Part print with two shaded views. Sizes in mm from the minimum x, y, z corner. Round coordinates to 2 decimals unless told otherwise and drop trailing zeros. Loops run counter-clockwise (first coordinate to the right, second up) from the corner with the lowest first, then second, coordinate; pieces in that order, holes last.
(1) Cut at B-B on x = 25. List the corners of the cut face in (y, z), then the cut area to 3 significant figures.
(2) Cut at D-D on z = 18.95. List the corners of the cut face in (x, y) (1 decimal).
(3) Flat gauge pins, fed straight in: pin 1 (6 mm diameter, centred on y = 13, z = 25.5, fed in from -X); pin 2 (6 mm diameter, centred on y = 26, z = 11, fed in from +X); pin 3 (1 mm diameter, centred on y = 9, z = 19, fed in from +X) (1 decimal); pin 4 (17.5 mm diameter, centred on x = 18.5, y = 15.5, fed in from -Z). Where does each tip first touch, or does it go through?
(4) Mould opens along Y. For the marked faces 1 and 2 say: +Y half, -Y half, draft (parallel to the pull), parting line (faces both ways), or undercut.
(5) Cut at A-A on y = 30. List the corners of the cut face in (x, z).
(6) Cut at C-C on z = 31.5. List the corners of the cut face in (x, y).
(7) Probe probe 1 along Y at (x, z) = (30, 11.5); probe 2 along Y at (x, z) = (30, 1); probe 3 along Z at (x, y) = (23.5, 2.5). List the from-to ranges inside material, lowest first.
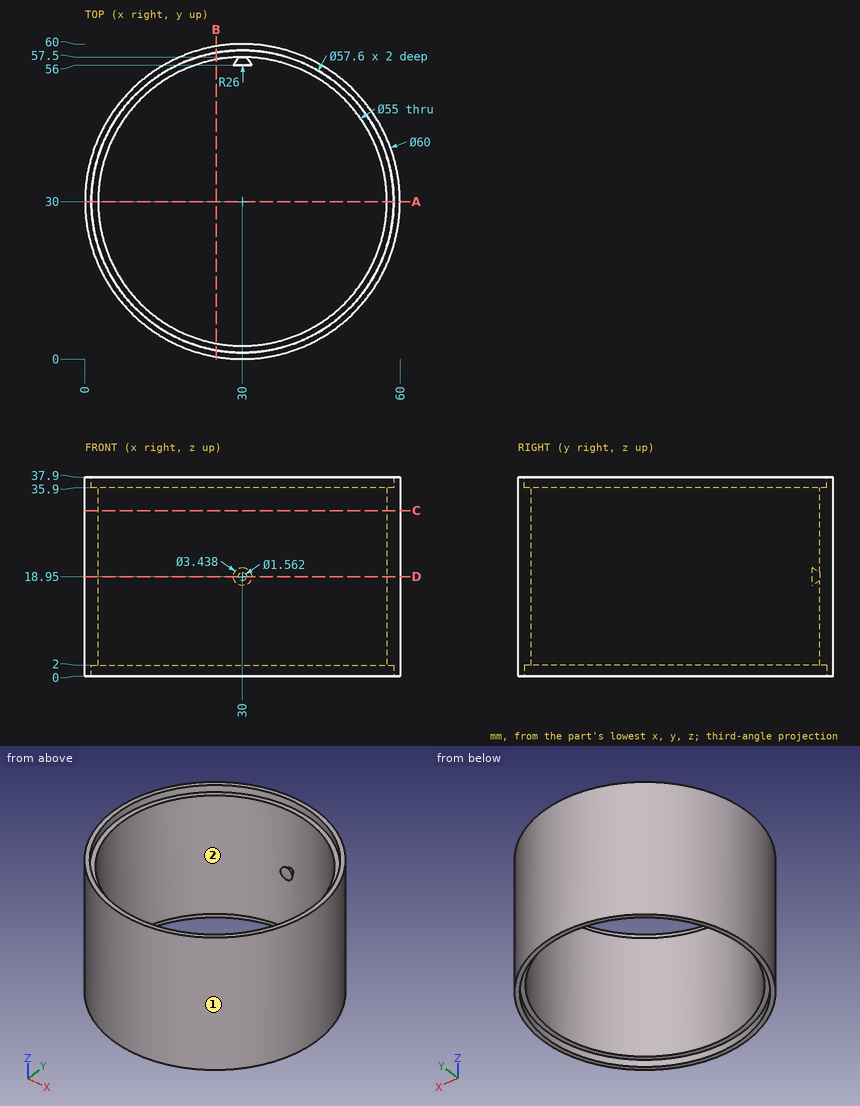
Final values:
1. outline: (0.42, 0) - (1.64, 0) - (1.64, 2) - (2.96, 2) - (2.96, 35.9) - (1.64, 35.9) - (1.64, 37.9) - (0.42, 37.9) - close; (57.04, 2) - (58.36, 2) - (58.36, 0) - (59.58, 0) - (59.58, 37.9) - (58.36, 37.9) - (58.36, 35.9) - (57.04, 35.9) - close
1. area: 182 mm2
2. outline: circle Ø60 at (30, 30); hole (28.2, 55.9) - (29.2, 57.5) arc R27.5 ccw (long way) to (30.8, 57.5) - (31.8, 55.9) arc R26 ccw to start
3. pin 1: stops at x = 3.47
3. pin 2: stops at x = 59.98
3. pin 3: stops at x = 51.9
3. pin 4: passes through
4. face 1: parting line
4. face 2: undercut
5. outline: (0, 0) - (1.2, 0) - (1.2, 2) - (2.5, 2) - (2.5, 35.9) - (1.2, 35.9) - (1.2, 37.9) - (0, 37.9) - close; (57.5, 2) - (58.8, 2) - (58.8, 0) - (60, 0) - (60, 37.9) - (58.8, 37.9) - (58.8, 35.9) - (57.5, 35.9) - close
6. outline: circle Ø60 at (30, 30); hole circle Ø55 at (30, 30)
7. probe 1: y = 0 to 2.5, 57.5 to 60
7. probe 2: y = 0 to 1.2, 58.8 to 60
7. probe 3: z = 2 to 35.9
